Check sheet for the modelled part. Datum: model origin and axes. Units: mm. Face numbers are marked on the shaded views. A direction names the side the tool comes from. Give positions to 0.01 mm unless a question says otherwise; leave off trailing zeros. Write each loop counter-clockwise with the first axis right and the second up, starting at its lowest first coordinate (ties: lowest second). Pieces come first, ordered by that corner, then holes. Notation, with made-up numbers: M 20.25,82.25 L 39.25,82.25 A10 cw 39.25,96.25 Z; hole C 62,-16.75 d10. An arc over 180 degrees is marked long. Write item = value, one per line. Start each with the question number.
1) Scan lines: L1, parallel to Y at x = 23, z = 8.5; L2, parallel to X at y = 31.5, z = 7.75; L3, parallel to Y at x = -21.5, z = 9.5. Record each from-to range of solid material in increasing order.
2) Set-up check for the marked faces 1 and 2: record each of +Z, -Z, +X, -X, +Y, -Y from which the full face is reachable in a straight line by a thin tool's end or side.
3) Sectioned sample at A-A, the plane y = 17. Record the cut outline in (x, z), then the cut area to 3 significant figures.
4) Gauge pin test, flat ends, axial feed: pin 1 (22.5 mm diameter, centred on x = -1.5, y = 13.5, fed in from +Z); pin 2 (1.5 mm diameter, centred on x = -1, z = 1.5, fed in from +Y); pin 3 (1.1 mm diameter, centred on x = -42, z = 9.5, fed in from -Y). Record the tip position at first contact, or that the pin passes through.
from build123d import *

# Parameters (mm, degrees)
IZIM1_W                     = 80
IZIM1_H                     = 130
IZIM1_W_2                   = 76.8
IZIM1_H_2                   = 126.8
IZIM1_W_3                   = 75.2
IZIM1_H_3                   = 125.2
IZIM1_R                     = 1
IZIM1_W_4                   = 20
IZIM1_H_4                   = 16
IZIM1_W_5                   = 4.8
IZIM1_H_5                   = 1.5
Y_KSEKLIK_EKSTR_ZYON1_DEPTH = 9
IZIM1_3_W                   = 4.8
IZIM1_3_H                   = 1.5
Y_KSEKLIK_EKSTR_ZYON2_DEPTH = 10.4
IZIM1_4_W                   = 76.8
IZIM1_4_H                   = 126.8
IZIM1_4_W_2                 = 75.2
IZIM1_4_H_2                 = 125.2
Y_KSEKLIK_EKSTR_ZYON3_DEPTH = 9.8
Y_KSEKLIK_EKSTR_ZYON4_DEPTH = 3
KES_EKSTR_ZYON1_DEPTH       = 52
KES_EKSTR_ZYON1_DEPTH_BACK  = 12
KES_EKSTR_ZYON2_DEPTH       = 42
KES_EKSTR_ZYON2_DEPTH_BACK  = 2


with BuildPart() as part:
    # izim1 → Y_kseklik-Ekstr_zyon1 (new body)
    # profile 1 of 4: a face of its own
    with BuildSketch(Plane.XY):
        with Locations((-13.05110417, -1.285301478)):
            Rectangle(IZIM1_W, IZIM1_H)
        with Locations((-13.05110417, -1.285301478)):
            Rectangle(IZIM1_W_2, IZIM1_H_2, mode=Mode.SUBTRACT)
    # profile 2 of 4: a face of its own
    with BuildSketch(Plane.XY):
        with Locations((-13.05110417, -1.285301478)):
            Rectangle(IZIM1_W_3, IZIM1_H_3)
        with Locations((-48.05110417, -1.285301478)):
            Circle(IZIM1_R, mode=Mode.SUBTRACT)
        with Locations((-48.05110417, -59.835301478)):
            Circle(IZIM1_R, mode=Mode.SUBTRACT)
        with Locations((-13.05110417, -59.835301478)):
            Circle(IZIM1_R, mode=Mode.SUBTRACT)
        with Locations((21.94889583, -59.835301478)):
            Circle(IZIM1_R, mode=Mode.SUBTRACT)
        with Locations((21.94889583, -1.285301478)):
            Circle(IZIM1_R, mode=Mode.SUBTRACT)
        with Locations((-13.05110417, 57.264698522)):
            Circle(IZIM1_R, mode=Mode.SUBTRACT)
        with Locations((21.94889583, 57.264698522)):
            Circle(IZIM1_R, mode=Mode.SUBTRACT)
        with Locations((-48.05110417, 57.264698522)):
            Circle(IZIM1_R, mode=Mode.SUBTRACT)
        Polygon((-49.05110417, 1.164698522), (-49.05110417, 54.814698522), (-45.60110417, 54.814698522), (-45.60110417, 59.714698522), (-15.50110417, 59.714698522), (-15.50110417, 54.814698522), (-10.60110417, 54.814698522), (-10.60110417, 59.714698522), (19.49889583, 59.714698522), (19.49889583, 54.814698522), (22.94889583, 54.814698522), (22.94889583, 1.164698522), (19.49889583, 1.164698522), (19.49889583, -3.735301478), (22.94889583, -3.766968147), (22.94889583, -57.385301478), (19.49889583, -57.385301478), (19.49889583, -62.285301478), (-10.60110417, -62.285301478), (-10.60110417, -57.385301478), (-15.50110417, -57.385301478), (-15.50110417, -62.285301478), (-45.60110417, -62.285301478), (-45.60110417, -57.385301478), (-49.05110417, -57.385301478), (-49.05110417, -3.735301478), (-45.60110417, -3.735301478), (-45.60110417, 1.164698522), align=None, mode=Mode.SUBTRACT)
    # profile 3 of 4: a face of its own
    with BuildSketch(Plane.XY):
        with Locations((16.94889583, 71.714698522)):
            Rectangle(IZIM1_W_4, IZIM1_H_4)
        with Locations((15.44889583, 65.464698522)):
            Rectangle(IZIM1_W_5, IZIM1_H_5, mode=Mode.SUBTRACT)
        with Locations((15.44889583, 77.964698522)):
            Rectangle(IZIM1_W_5, IZIM1_H_5, mode=Mode.SUBTRACT)
        with Locations((22.94889583, 67.714698522)):
            Circle(IZIM1_R, mode=Mode.SUBTRACT)
        with Locations((22.94889583, 75.714698522)):
            Circle(IZIM1_R, mode=Mode.SUBTRACT)
    # profile 4 of 4: a face of its own
    with BuildSketch(Plane.XY):
        with Locations((-43.05110417, 71.714698522)):
            Rectangle(IZIM1_W_4, IZIM1_H_4)
        with Locations((-49.05110417, 67.714698522)):
            Circle(IZIM1_R, mode=Mode.SUBTRACT)
        with Locations((-49.05110417, 75.714698522)):
            Circle(IZIM1_R, mode=Mode.SUBTRACT)
        with Locations((-41.55110417, 65.464698522)):
            Rectangle(IZIM1_W_5, IZIM1_H_5, mode=Mode.SUBTRACT)
        with Locations((-41.55110417, 77.964698522)):
            Rectangle(IZIM1_W_5, IZIM1_H_5, mode=Mode.SUBTRACT)
    extrude(amount=Y_KSEKLIK_EKSTR_ZYON1_DEPTH)

    # izim1_3 → Y_kseklik-Ekstr_zyon2 (add)
    with BuildSketch(Plane.XY):
        with Locations((15.44889583, 65.464698522)):
            Rectangle(IZIM1_3_W, IZIM1_3_H)
        with Locations((15.44889583, 77.964698522)):
            Rectangle(IZIM1_3_W, IZIM1_3_H)
        with Locations((-41.55110417, 77.964698522)):
            Rectangle(IZIM1_3_W, IZIM1_3_H)
        with Locations((-41.55110417, 65.464698522)):
            Rectangle(IZIM1_3_W, IZIM1_3_H)
    extrude(amount=Y_KSEKLIK_EKSTR_ZYON2_DEPTH)

    # izim1_4 → Y_kseklik-Ekstr_zyon3 (add)
    with BuildSketch(Plane.XY):
        with Locations((-13.05110417, -1.285301478)):
            Rectangle(IZIM1_4_W, IZIM1_4_H)
        with Locations((-13.05110417, -1.285301478)):
            Rectangle(IZIM1_4_W_2, IZIM1_4_H_2, mode=Mode.SUBTRACT)
    extrude(amount=Y_KSEKLIK_EKSTR_ZYON3_DEPTH)

    # izim1_5 → Y_kseklik-Ekstr_zyon4 (add)
    with BuildSketch(Plane.XY):
        Polygon((-49.05110417, 54.814698522), (-45.60110417, 54.814698522), (-45.60110417, 59.714698522), (-15.50110417, 59.714698522), (-15.50110417, 54.814698522), (-10.60110417, 54.814698522), (-10.60110417, 59.714698522), (19.49889583, 59.714698522), (19.49889583, 54.814698522), (22.94889583, 54.814698522), (22.94889583, 1.164698522), (19.49889583, 1.164698522), (19.49889583, -3.735301478), (22.94889583, -3.766968147), (22.94889583, -57.385301478), (19.49889583, -57.385301478), (19.49889583, -62.285301478), (-10.60110417, -62.285301478), (-10.60110417, -57.385301478), (-15.50110417, -57.385301478), (-15.50110417, -62.285301478), (-45.60110417, -62.285301478), (-45.60110417, -57.385301478), (-49.05110417, -57.385301478), (-49.05110417, -3.735301478), (-45.60110417, -3.735301478), (-45.60110417, 1.164698522), (-49.05110417, 1.164698522), align=None)
    extrude(amount=Y_KSEKLIK_EKSTR_ZYON4_DEPTH)

    # izim2 → Kes-Ekstr_zyon1 (cut, two sides: drawn at the far end of the back side and taken through both)
    with BuildSketch(Plane.ZY.offset(-6.94889583).offset(-KES_EKSTR_ZYON1_DEPTH_BACK)):
        with BuildLine():
            Line((9, 67.714698522), (9, 75.714698522))
            ThreePointArc((9, 75.714698522), (5, 71.714698522), (9, 67.714698522))
        make_face()
    extrude(amount=KES_EKSTR_ZYON1_DEPTH + KES_EKSTR_ZYON1_DEPTH_BACK, mode=Mode.SUBTRACT)

    # izim2_3 → Kes-Ekstr_zyon2 (cut, two sides: drawn at the far end of the back side and taken through both)
    with BuildSketch(Plane.ZY.offset(-6.94889583).offset(-KES_EKSTR_ZYON2_DEPTH_BACK)):
        with BuildLine():
            Line((9, 75.714698522), (9, 77.714698522))
            ThreePointArc((9, 77.714698522), (3, 71.714698522), (9, 65.714698522))
            Line((9, 65.714698522), (9, 67.714698522))
            ThreePointArc((9, 67.714698522), (5, 71.714698522), (9, 75.714698522))
        make_face()
    extrude(amount=KES_EKSTR_ZYON2_DEPTH + KES_EKSTR_ZYON2_DEPTH_BACK, mode=Mode.SUBTRACT)


solid = part.part
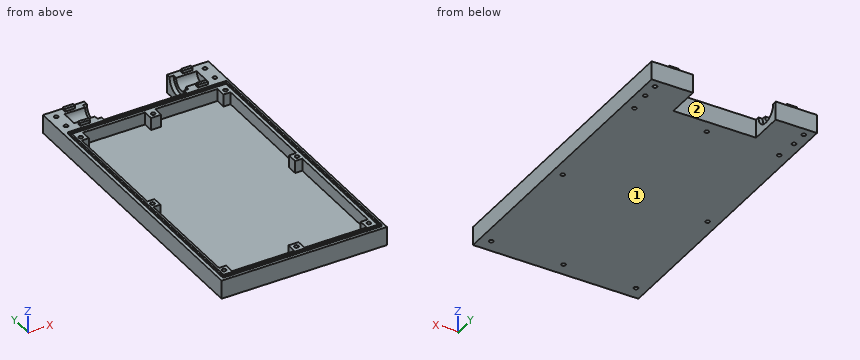
Data:
q1.L1 = -66.29 to 66.72, 68.71 to 74.72, 76.71 to 79.71
q1.L2 = -53.05 to -49.05, 22.95 to 26.95
q1.L3 = -64.69 to -63.89, 61.31 to 62.11
q2.face_1 = -Z, +X, -X, +Y, -Y
q2.face_2 = +Z, -Z, +Y
q3.outline = M -53.05,0 L 26.95,0 L 26.95,9 L 25.35,9 L 25.35,9.8 L 24.55,9.8 L 24.55,9 L 22.95,9 L 22.95,3 L -49.05,3 L -49.05,9 L -50.65,9 L -50.65,9.8 L -51.45,9.8 L -51.45,9 L -53.05,9 Z
q3.area = 289 mm2
q4.pin_1 = 3
q4.pin_2 = 63.71
q4.pin_3 = -66.29
